Autodesk Inventor part; units mm, degrees
ref_plane "YZ Plane" through (0, 0, 0) normal (1, 0, 0) x (0, 1, 0)
ref_plane "XZ Plane" through (0, 0, 0) normal (0, 1, 0) x (-1, 0, 0)
ref_plane "XY Plane" through (0, 0, 0) normal (0, 0, 1) x (1, 0, 0)
sketch "Sketch1" plane through (0, 0, 0) normal (1, 0, 0) x (0, 1, 0)
  circle A0 centre (0, 0) radius 90 construction
  circle A1 centre (0, 0) radius 12.5
  circle A2 centre (0, 0) radius 25
  line L0 (77.9423, 45) -> (77.9423, -45) construction
  line L1 (-8.0516, 23.668) -> (75.5268, 52.1004)
  circle A3 centre (77.9423, 45) radius 2.2
  circle A4 centre (77.9423, 45) radius 7.5
  line L2 (82.1544, 38.7945) -> (25, 0)
  line L3 (0, 0) -> (51.9077, 0)
  line L4 (-8.0516, -23.668) -> (75.5268, -52.1004)
  circle A5 centre (77.9423, -45) radius 2.2
  circle A6 centre (77.9423, -45) radius 7.5
  line L5 (82.1544, -38.7945) -> (25, 0)
  point P0 (77.9423, 0)
  dimension "d0" = 180
  dimension "d1" = 25
  dimension "d2" = 50
  dimension "d3" = 90
  dimension "d4" = 4.4
  dimension "d5" = 15
extrude "Extrusion1" add sketch "Sketch1" along normal blind 14
fillet "Fillet1" radius 5 1 edges at (7, 25, 0)
sketch "Sketch2" plane through (14, 0, 0) normal (1, 0, 0) x (0, 0, -1)
  circle A0 centre (0, 0) radius 12.5
  circle A1 centre (0, 0) radius 21.15
  dimension "d9" = 42.3
extrude "Extrusion2" cut sketch "Sketch2" against normal blind 12
sketch "Sketch3" plane through (14, 0, 0) normal (1, 0, 0) x (0, 0, -1)
  circle A0 centre (0, 0) radius 21.15
  arc A1 (-38.7945, 82.1544) -> (-52.1004, 75.5268) centre (-45, 77.9423) ccw
  line L0 (-52.1004, 75.5268) -> (-23.668, -8.0516)
  arc A2 (-23.668, -8.0516) -> (23.668, -8.0516) centre (0, 0) ccw
  line L1 (23.668, -8.0516) -> (52.1004, 75.5268)
  arc A3 (52.1004, 75.5268) -> (38.7945, 82.1544) centre (45, 77.9423) ccw
  line L2 (38.7945, 82.1544) -> (4.137, 31.0949)
  arc A4 (-4.137, 31.0949) -> (4.137, 31.0949) centre (0, 33.9029) ccw
  line L3 (-4.137, 31.0949) -> (-38.7945, 82.1544)
  circle A5 centre (45, 77.9423) radius 2.2
  circle A6 centre (-45, 77.9423) radius 2.2
  circle A7 centre (-45, 77.9423) radius 7.5
  circle A8 centre (45, 77.9423) radius 7.5
  point P0 (38.7945, 82.1544)
  point P1 (52.1004, 75.5268)
  point P2 (-52.1004, 75.5268)
extrude "Extrusion3" add sketch "Sketch3" along normal blind 6 contours A7 A1 | A3 A8
sketch "Sketch4" plane through (0, 0, 0) normal (-1, 0, 0) x (0, 0, 1)
  arc A0 (52.1004, 75.5268) -> (38.7945, 82.1544) centre (45, 77.9423) ccw
  line L0 (4.137, 31.0949) -> (38.7945, 82.1544)
  arc A1 (-4.137, 31.0949) -> (4.137, 31.0949) centre (0, 33.9029) ccw
  line L1 (-38.7945, 82.1544) -> (-4.137, 31.0949)
  arc A2 (-38.7945, 82.1544) -> (-52.1004, 75.5268) centre (-45, 77.9423) ccw
  line L2 (-23.668, -8.0516) -> (-52.1004, 75.5268)
  arc A3 (-23.668, -8.0516) -> (23.668, -8.0516) centre (0, 0) ccw
  line L3 (52.1004, 75.5268) -> (23.668, -8.0516)
  circle A4 centre (-45, 77.9423) radius 2.2
  circle A5 centre (45, 77.9423) radius 2.2
  circle A6 centre (0, 0) radius 12.5
  circle A7 centre (-45, 77.9423) radius 4.2
  circle A8 centre (45, 77.9423) radius 4.2
  dimension "d14" = 8.4
extrude "Extrusion4" cut sketch "Sketch4" against normal blind 9 contours A4 | A5 | A7 | A8
sketch "Sketch5" plane through (0, 0, 0) normal (-1, 0, 0) x (0, 0, 1)
  circle A0 centre (45, 77.9423) radius 4.2
  circle A1 centre (-45, 77.9423) radius 4.2
  arc A2 (52.1004, 75.5268) -> (38.7945, 82.1544) centre (45, 77.9423) ccw
  line L0 (4.137, 31.0949) -> (38.7945, 82.1544)
  arc A3 (-4.137, 31.0949) -> (4.137, 31.0949) centre (0, 33.9029) ccw
  line L1 (-38.7945, 82.1544) -> (-4.137, 31.0949)
  arc A4 (-38.7945, 82.1544) -> (-52.1004, 75.5268) centre (-45, 77.9423) ccw
  line L2 (-23.668, -8.0516) -> (-52.1004, 75.5268)
  arc A5 (-23.668, -8.0516) -> (23.668, -8.0516) centre (0, 0) ccw
  line L3 (52.1004, 75.5268) -> (23.668, -8.0516)
  circle A6 centre (0, 0) radius 12.5
  line L4 (-30, 51.9615) -> (30, 51.9615) construction
  line L5 (-45, 77.9423) -> (0, 0)
  circle A7 centre (45, 77.9423) radius 2.2
  line L6 (0, 0) -> (45, 77.9423)
  circle A8 centre (-30, 51.9615) radius 1.65
  circle A9 centre (30, 51.9615) radius 1.65
  point P0 (0, 51.9615)
  dimension "d17" = 60
  dimension "d18" = 3.3
  dimension "d19" = 3.3
extrude "Extrusion5" cut sketch "Sketch5" against normal through all contours A8 L5 | L5 A8 | A9 L6 | L6 A9
properties part number "SOPORTE_RODAMIENTO" material "Steel, Mild, Welded"
Work out the finished part from the listing and answer in its coordinate system (mm). A direction names the side the tool comes from. Give positions to 0.01 mm unless a question says otherwise; leave off trailing zeros. Order: outer loops, then holes, each group sorted by start corner. A loop starts at its lowest first (then second) coordinate and runs counter-clockwise, first axis right, second up. Notation, with made-up numbers: M 21.5,-24.75 L 73.5,-24.75 A15 ccw 73.5,-5.75 Z; hole C 4.25,-37 d7. An arc over 180 degrees is marked long. Return JSON: item names as keys, results as strings.
1) Section D-D, the plane y = 17 is taken. Write down the section's boundary in (x, z), plus the area to 3 significant figures.
Resolved:
{"outline": "M 0,-32.19 L 14,-32.19 L 14,-12.58 L 2,-12.58 L 2,12.58 L 14,12.58 L 14,32.19 L 0,32.19 Z", "area": "599 mm^2"}
2) Section B-B, the plane y = 62 is taken. Write down the section's boundary in (x, z).
Resolved:
{"outline": "M 0,-47.5 L 14,-47.5 L 14,-25.11 L 0,-25.11 Z; M 0,25.11 L 14,25.11 L 14,47.5 L 0,47.5 Z"}
3) Section C-C, the plane x = 5.75 is taken. Write down the section's boundary in (y, z).
Resolved:
{"outline": "M -8.05,-23.67 L 75.53,-52.1 A7.5 ccw 82.15,-38.79 L 31.09,-4.14 A5 cw 31.09,4.14 L 82.15,38.79 A7.5 ccw 75.53,52.1 L -8.05,23.67 A25 ccw Z; hole C 0,0 d42.3; hole C 51.96,-30 d3.3; hole C 51.96,30 d3.3; hole C 77.94,-45 d8.4; hole C 77.94,45 d8.4"}
4) Straight lines are drawn through the part: line 1 along Z through (x, y) = (2, 77); line 2 along Z through (x, y) = (1.5, 78); line 3 along Z through (x, y) = (4, 59.5). For each, find the intervals that lie inside material, in ascending order. Write a range as [from, to].
Resolved:
{"line 1": "[-52.44, -49.09], [-40.91, -35.3], [35.3, 40.91], [49.09, 52.44]", "line 2": "[-52.5, -49.2], [-40.8, -35.97], [35.97, 40.8], [49.2, 52.5]", "line 3": "[-46.65, -23.42], [23.42, 46.65]"}
5) For a pull along Z with two mould halves and no side action, classify faces 6 (the flat face through (6.902, 56.982, 21.708)), 7 (the cylindrical face through (7, -25, 0)), 8 (the flat face through (20, 76, 43)) as +Z half, -Z half, draft (parallel to the pull), parting line (faces both ways), or undercut.
Resolved:
{"face 6": "undercut", "face 7": "parting line", "face 8": "draft"}
6) Each of these flat-tipped pins is pushed along its axis until it touches: pin 1 (3.5 mm diameter, centred on y = 77.94, z = 45, fed in from -X); pin 2 (5 mm diameter, centred on x = 6.5, y = -2, fed in from -Z); pin 3 (3 mm diameter, centred on y = 39.5, z = -17, fed in from +X); pin 4 (3 mm diameter, centred on x = 6, y = 71.5, fed in from -Z). Where does it stop, or does it pass through?
Resolved:
{"pin 1": "through", "pin 2": "z = -26.58", "pin 3": "x = 14", "pin 4": "z = -51.24"}
7) Section A-A, the plane z = 0 is taken. Write down the section's boundary in (x, y), plus the area to 3 significant figures.
Resolved:
{"outline": "M 0,-25 L 14,-25 L 14,-21.15 L 2,-21.15 L 2,-12.5 L 0,-12.5 Z; M 0,12.5 L 2,12.5 L 2,21.15 L 14,21.15 L 14,28.9 L 0,28.9 Z", "area": "197 mm^2"}
8) A tool of negligible diameter and unlimited length cuts with its end or side. For faces 1 (the flat face through (20, 76, -47)), 2 (the cylindrical face through (16.96, 71.31, 41.5)), 3 (the flat face through (6.902, 56.982, -21.708)), 4 (the flat face through (9, 76, -43)), 5 (the cylindrical face through (6.9, 53.6, -30.2)), from which of +Z, -Z, +X, -X, +Y, -Y can it reach the whole face along a straight path? Write none if from no direction.
Resolved:
{"face 1": "+Z, -Z, +X, +Y, -Y", "face 2": "+X", "face 3": "+X, -X, +Y", "face 4": "-X", "face 5": "+X, -X"}
